Geometry check sheet. Reference: the model listing, model coordinates, mm. Face numbers are marked on the shaded views. A direction names the side the tool comes from. Coordinates: 2 decimals unless noted, no trailing zeros. Write each loop counter-clockwise with the first axis right and the second up, starting at its lowest first coordinate (ties: lowest second). Pieces come first, ordered by that corner, then holes. Notation, with made-up numbers: (74.5, -35.75) -> (123.5, -35.75) arc R24 ccw to (123.5, -16.75) -> close; hole circle Ø10 at (-20, -9.5). An arc over 180 degrees is marked (long way). One line per question, with ' | ' between items.
from build123d import *

# Parameters (mm, degrees)
SKETCH1_R           = 7
BOSS_EXTRUDE1_DEPTH = 25
BOSS_EXTRUDE2_START = 12
BOSS_EXTRUDE2_DEPTH = 24
SKETCH1_4_R         = 7.000000000000007
BOSS_EXTRUDE3_DEPTH = 12
BOSS_EXTRUDE6_START = 36
SKETCH1_7_R         = 7.000000000000007
BOSS_EXTRUDE6_DEPTH = 12
SHELL7_T            = -1
BOSS_EXTRUDE7_DEPTH = 36
SKETCH2_R           = 9.695738558294309
CUT_EXTRUDE2_DEPTH  = 93.13576938409969


with BuildPart() as part:
    # Sketch1 → Boss-Extrude1 (new body)
    with BuildSketch(Plane.XY):
        Polygon((-72, -1.421e-14), (-72, -18.000000000000014), (-64.99999999999997, -25.000000000000014), (-38, -25.000000000000007), (-38.00000000000001, 3.4734603858306787), (-57.99999999999999, 6.999999999999986), (-65.00000000000001, 6.999999999999986), align=None)
        with Locations((-57.99999999999999, -11.000000000000014)):
            Circle(SKETCH1_R, mode=Mode.SUBTRACT)
    extrude(amount=BOSS_EXTRUDE1_DEPTH)

    # Sketch1_4 → Boss-Extrude3 (add)
    # profile 1 of 2: a face of its own
    with BuildSketch(Plane.XY):
        with BuildLine():
            ThreePointArc((-24.763063450975714, 4.344294617344023), (-13.815737017505185, -12.419294771345367), (3.764705882352942, -22.000000000000004))
            Line((3.764705882352942, -22), (14, -10))
            Line((14, -9.999999999999998), (13.999999999999998, 9.000000000000002))
            Line((13.999999999999998, 9.000000000000002), (8.999999999999979, 14))
            Line((8.999999999999979, 14), (-15.000000000000004, 14))
            ThreePointArc((-15.000000000000004, 14), (-18.97875565666663, 8.259333620533186), (-24.76306345097571, 4.344294617344016))
        make_face()
        Circle(SKETCH1_4_R, mode=Mode.SUBTRACT)
    # profile 2 of 2: a face of its own
    with BuildSketch(Plane.XY):
        with BuildLine():
            Line((-38.00000000000001, 3.4734603858306787), (-38, -25.000000000000014))
            Line((-38, -25.000000000000007), (-32.424461088659314, -25.000000000000007))
            Line((-32.424461088659314, -25.00000000000001), (1.2058823529411669, -25.00000000000001))
            Line((1.2058823529411704, -25.00000000000001), (3.764705882352942, -22))
            ThreePointArc((3.764705882352942, -22.000000000000004), (-13.815737017505185, -12.419294771345367), (-24.763063450975714, 4.344294617344023))
            ThreePointArc((-24.76306345097571, 4.344294617344016), (-30.106088890163186, 2.9001323723087005), (-35.63861916422293, 3.0570852327552736))
            Line((-35.63861916422293, 3.057085232755278), (-38.00000000000001, 3.4734603858306823))
        make_face()
    extrude(amount=BOSS_EXTRUDE3_DEPTH)

    # Sketch1_8 → Boss-Extrude7 (add)
    with BuildSketch(Plane.XY):
        with BuildLine():
            Line((1.2058823529411669, -25.00000000000001), (-32.424461088659314, -25.00000000000001))
            ThreePointArc((-32.424461088659314, -25.000000000000007), (-29.159225307604235, -26.213413767769495), (-27.478822347247476, -29.26470588235295))
            ThreePointArc((-27.47882234724748, -29.264705882352946), (-25.141992144084263, -37.11567206097118), (-20.70301994726548, -44.000000000000014))
            Line((-20.70301994726548, -44.000000000000014), (-14.999999999999996, -44.00000000000001))
            Line((-14.999999999999996, -44.00000000000001), (1.2058823529411704, -25.00000000000001))
        make_face()
    extrude(amount=BOSS_EXTRUDE7_DEPTH)


with BuildPart() as body_2:
    # Sketch1_3 → Boss-Extrude2 (new body)
    with BuildSketch(Plane.XY.offset(BOSS_EXTRUDE2_START)):
        with BuildLine():
            Line((-38.00000000000001, 3.4734603858306787), (-38, -25.000000000000014))
            Line((-38, -25.000000000000007), (-32.424461088659314, -25.000000000000007))
            Line((-32.424461088659314, -25.00000000000001), (1.2058823529411669, -25.00000000000001))
            Line((1.2058823529411704, -25.00000000000001), (3.764705882352942, -22))
            ThreePointArc((3.764705882352942, -22.000000000000004), (-13.815737017505185, -12.419294771345367), (-24.763063450975714, 4.344294617344023))
            ThreePointArc((-24.76306345097571, 4.344294617344016), (-30.106088890163186, 2.9001323723087005), (-35.63861916422293, 3.0570852327552736))
            Line((-35.63861916422293, 3.057085232755278), (-38.00000000000001, 3.4734603858306823))
        make_face()
    extrude(amount=BOSS_EXTRUDE2_DEPTH)

    # Sketch1_7 → Boss-Extrude6 (add)
    # profile 1 of 2: a face of its own
    with BuildSketch(Plane.XY.offset(BOSS_EXTRUDE6_START)):
        with BuildLine():
            ThreePointArc((-24.763063450975714, 4.344294617344023), (-13.815737017505185, -12.419294771345367), (3.764705882352942, -22.000000000000004))
            Line((3.764705882352942, -22), (14, -10))
            Line((14, -9.999999999999998), (13.999999999999998, 9.000000000000002))
            Line((13.999999999999998, 9.000000000000002), (8.999999999999979, 14))
            Line((8.999999999999979, 14), (-15.000000000000004, 14))
            ThreePointArc((-15.000000000000004, 14), (-18.97875565666663, 8.259333620533186), (-24.76306345097571, 4.344294617344016))
        make_face()
        Circle(SKETCH1_7_R, mode=Mode.SUBTRACT)
    # profile 2 of 2: a face of its own
    with BuildSketch(Plane.XY.offset(BOSS_EXTRUDE6_START)):
        with BuildLine():
            Line((-38.00000000000001, 3.4734603858306787), (-38, -25.000000000000014))
            Line((-38, -25.000000000000007), (-32.424461088659314, -25.000000000000007))
            Line((-32.424461088659314, -25.00000000000001), (1.2058823529411669, -25.00000000000001))
            Line((1.2058823529411704, -25.00000000000001), (3.764705882352942, -22))
            ThreePointArc((3.764705882352942, -22.000000000000004), (-13.815737017505185, -12.419294771345367), (-24.763063450975714, 4.344294617344023))
            ThreePointArc((-24.76306345097571, 4.344294617344016), (-30.106088890163186, 2.9001323723087005), (-35.63861916422293, 3.0570852327552736))
            Line((-35.63861916422293, 3.057085232755278), (-38.00000000000001, 3.4734603858306823))
        make_face()
    extrude(amount=BOSS_EXTRUDE6_DEPTH)

    # Shell7
    shell7_openings = [body_2.faces().sort_by_distance(p)[0] for p in [
        (-12.583479215, -7.183735209, 48),
    ]]
    offset(amount=SHELL7_T, openings=shell7_openings, kind=Kind.INTERSECTION)


with BuildPart() as part_1:
    add(part.part)

    # Combine1: union body 2
    add(body_2.part)

    # Sketch2 → Cut-Extrude2 (cut, through all)
    with BuildSketch(Plane.XY.offset(37)):
        Circle(SKETCH2_R)
    extrude(amount=CUT_EXTRUDE2_DEPTH, mode=Mode.SUBTRACT)


solid = part_1.part
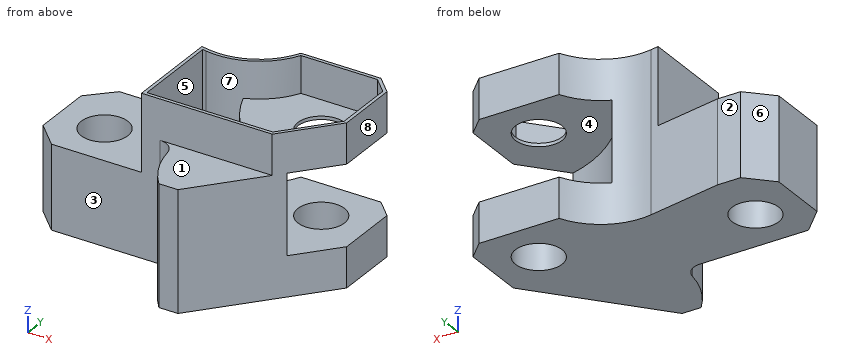
1. Mould release check, pull along X, two halves, no side actions. Record for the marked faces 6, 7 and 8: released by +X, released by -X, zero draft, split by the parting line, or undercut.
Worked answers:
face 6: released by -X | face 7: undercut | face 8: released by +X
2. Go/stop test with flat-tipped pins: P1, Ø6, axis at x = -33, z = 19.5, coming from the -Y side; P2, Ø7.5, axis at x = -60.5, z = 12.5, coming from the +Y side; P3, Ø2, axis at x = -0.5, z = 21, coming from the +Y side; P4, Ø5, axis at x = 2, y = 2, coming from the -Z side. Record where each tip stops, or that it passes through.
Worked answers:
P1: y = -25.63 | P2: y = 7 | P3: y = -20.26 | P4: through
3. Cross-section at D-D on z = 18.5. Record the boundary of the cut face in (x, y).
Worked answers:
outline: (-72, -18) -> (-65, -25) -> (-32.42, -25) arc R5 cw to (-27.48, -29.26) arc R29 ccw to (-20.7, -44) -> (-15, -44) -> (3.76, -22) arc R41 cw to (-24.76, 4.34) arc R19 cw to (-35.64, 3.06) -> (-58, 7) -> (-65, 7) -> (-72, 0) -> close; hole circle Ø14 at (-58, -11); hole (-37, -24) -> (0.74, -24) -> (1.99, -22.54) arc R42 cw to (-25.35, 3.03) arc R20 cw to (-35.81, 2.07) -> (-37, 2.28) -> close
4. Cross-section at C-C on x = -53. Record the boundary of the cut face in (y, z), and give its area (3 significant figures).
Worked answers:
outline: (-25, 0) -> (-15.9, 0) -> (-15.9, 25) -> (-25, 25) -> close; (-6.1, 0) -> (6.12, 0) -> (6.12, 25) -> (-6.1, 25) -> close | area: 533 mm²
5. Material ranges on line 1 (Y direction, x = 0, z = 36.75); line 2 (X direction, y = -8.5, z = 22); line 3 (Z direction, x = -14.5, y = 1), recorded low to high. Write a range as from..to.
Worked answers:
line 1: -25..-24, -21.9..-7, 7..14 | line 2: -72..-64.54, -51.46..-37, -18.82..-17.54 | line 3: 0..12, 36..37
6. Tool access check on the marked faces 1, 2, 3, 4 and 5. Record the directions out of +Z, -Z, +X, -X, +Y, -Y that give a thin tool (end or side, any length) a straight path to the whole face; none if there is none.
Worked answers:
face 1: +Z, +X, -X, -Y | face 2: +Z, -Z, -X, +Y | face 3: +Z, -X, -Y | face 4: +X, +Y | face 5: +Z
7. Cross-section at A-A on y = -11. Record the boundary of the cut face in (x, z), and give its area (3 significant figures).
Worked answers:
outline: (-72, 0) -> (-65, 0) -> (-65, 25) -> (-72, 25) -> close; (-51, 0) -> (13.15, 0) -> (13.15, 12) -> (-15.28, 12) -> (-15.28, 36) -> (13.15, 36) -> (13.15, 48) -> (11.83, 48) -> (11.83, 37) -> (-16.66, 37) -> (-16.66, 13) -> (-37, 13) -> (-37, 48) -> (-38, 48) -> (-38, 25) -> (-51, 25) -> close | area: 1,250 mm²
8. Cross-section at B-B on z = 29. Record the boundary of the cut face in (x, y), and give its area (3 significant figures).
Worked answers:
outline: (-38, -25) -> (-32.42, -25) arc R5 cw to (-27.48, -29.26) arc R29 ccw to (-20.7, -44) -> (-15, -44) -> (3.76, -22) arc R41 cw to (-24.76, 4.34) arc R19 cw to (-35.64, 3.06) -> (-38, 3.47) -> close; hole (-37, -24) -> (0.74, -24) -> (1.99, -22.54) arc R42 cw to (-25.35, 3.03) arc R20 cw to (-35.81, 2.07) -> (-37, 2.28) -> close | area: 480 mm²
